Check sheet for the modelled part. Datum: model origin and axes. Units: mm. Face numbers are marked on the shaded views. Coordinates: 2 decimals unless noted, no trailing zeros. Write each loop counter-clockwise with the first axis right and the second up, starting at its lowest first coordinate (ties: lowest second). Pieces come first, ordered by that corner, then holes. Notation, with made-up numbers: (39.25, 33) - (98.25, 33) arc R33 ccw to (98.25, 68) - close; hole circle Ø3 at (-35.75, 27). An arc over 180 degrees is marked (long way). Write each question's results on one line, items separated by ' | '.
from build123d import *

# Parameters (mm, degrees)
SKETCH1_R           = 1.778
SKETCH1_R_2         = 1.55
SKETCH1_R_3         = 5
BOSS_EXTRUDE1_DEPTH = 6.35
FILLET1_R           = 10


with BuildPart() as part:
    # Sketch1 → Boss-Extrude1 (new body)
    with BuildSketch(Plane.XY):
        with BuildLine():
            Line((90.617041925, 17.461725961), (30, 25))
            Line((30, 25), (0, 25))
            Line((0, 25), (0, 0))
            Line((0, 0), (30, 0))
            Line((30, 0), (90.617033237, 7.538165184))
            ThreePointArc((90.617033237, 7.538165184), (95, 12.499941736), (90.617041925, 17.461725961))
        make_face()
        with Locations((24.779, 12.499946113)):
            Circle(SKETCH1_R, mode=Mode.SUBTRACT)
        with Locations((5.221, 12.499946113)):
            Circle(SKETCH1_R, mode=Mode.SUBTRACT)
        with Locations((90, 12.499946113)):
            Circle(SKETCH1_R_2, mode=Mode.SUBTRACT)
        with Locations((15, 12.499946113)):
            Circle(SKETCH1_R_3, mode=Mode.SUBTRACT)
    extrude(amount=BOSS_EXTRUDE1_DEPTH)

    # Fillet1
    fillet1_edges = [part.edges().sort_by_distance(p)[0] for p in [
        (0, 0, 3.175),
        (0, 25, 3.175),
    ]]
    fillet(fillet1_edges, radius=FILLET1_R)


solid = part.part
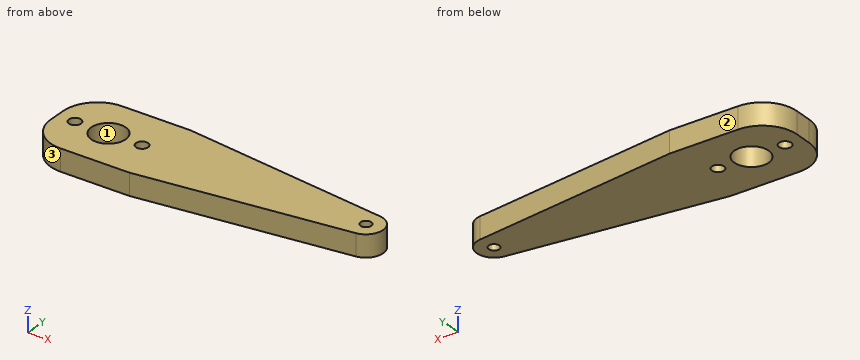
1. Sectioned sample at A-A (x = 15). Record the cut outline in (y, z).
Values follow:
outline: (0, 0) - (7.5, 0) - (7.5, 6.35) - (0, 6.35) - close; (17.5, 0) - (25, 0) - (25, 6.35) - (17.5, 6.35) - close
2. Sectioned sample at B-B (z = 3.75). Record the cut outline in (x, y), then the cut area to 3 significant figures.
Values follow:
outline: (0, 10) arc R10 ccw to (10, 0) - (30, 0) - (90.62, 7.54) arc R5 ccw to (90.62, 17.46) - (30, 25) - (10, 25) arc R10 ccw to (0, 15) - close; hole circle Ø3.56 at (5.22, 12.5); hole circle Ø10 at (15, 12.5); hole circle Ø3.56 at (24.78, 12.5); hole circle Ø3.1 at (90, 12.5) | area: 1,690 mm^2
3. Sectioned sample at D-D (x = 51.5). Record the cut outline in (y, z), then the cut area to 3 significant figures.
Values follow:
outline: (2.67, 0) - (22.33, 0) - (22.33, 6.35) - (2.67, 6.35) - close | area: 125 mm^2
4. Go/stop test with a flat-tipped pin: pin 1 (3 mm diameter, centred on x = 5.22, y = 12.5, fed in from +Z). Record where the tip stops, or that it passes through.
Values follow:
pin 1: passes through
5. Draft check along X on the marked faces 1, 2 and 3. Enter one of: pulls with the +X half, pulls with the -X half, needs draft (parallel to the pull), parting line crosses it, or undercut.
Values follow:
face 1: undercut | face 2: needs draft | face 3: pulls with the -X half
6. Material ranges on L1, parallel to Y at x = 15, z = 2.75; L2, parallel to Y at x = 90.5, z = 2.25; L3, parallel to X at y = 14.5, z = 1.5, recorded low to high. Write a range as [from, to].
Values follow:
L1: y = [0, 7.5], [17.5, 25] | L2: y = [7.52, 11.03], [13.97, 17.48] | L3: x = [0, 10.42], [19.58, 94.58]
7. Sectioned sample at C-C (x = 67). Record the cut outline in (y, z).
Values follow:
outline: (4.6, 0) - (20.4, 0) - (20.4, 6.35) - (4.6, 6.35) - close
